```python
from build123d import *

# Parameters (mm, degrees)
F1_DEPTH = 3.175
F2_W     = 6.985
F2_H     = 3.175
F3_DEPTH = 6.35
F5_DEPTH = 25.4
F6_DEPTH = 25.4
F7_DEPTH = 26.6192
F8_DEPTH = 26.6192


# Not quite as in the source:
# - a feature names something its author has since deleted; it is built from what else it names


with BuildPart() as f1:
    # F0 (on Top) → F1 (new body)
    with BuildSketch(Plane.XY):
        Polygon((0, 63.5), (0, 0), (15.875, 0), (15.875, 12.7), (12.065, 12.7), (12.065, 50.8), (15.875, 50.8), (15.875, 63.5), align=None)
        Polygon((15.875, 12.7), (15.875, 0), (31.75, 0), (31.75, 63.5), (15.875, 63.5), (15.875, 50.8), (19.685, 50.8), (19.685, 12.7), align=None)
    extrude(amount=F1_DEPTH)

    # F2 (on face) → F3 (join)
    with BuildSketch(Plane.XZ):
        with Locations((3.4925, 1.5875)):
            Rectangle(F2_W, F2_H)
        with Locations((28.2575, 1.5875)):
            Rectangle(F2_W, F2_H)
    extrude(amount=F3_DEPTH)

    # F4 (on face) → F5 (cut)
    with BuildSketch(Plane.XY.offset(3.175)):
        with BuildLine():
            ThreePointArc((5.29375, -4.35), (3.0318335149, -3.4130835149), (3.96875, -5.675))
            Line((3.96875, -5.675), (3.96875, -4.35))
            Line((3.96875, -4.35), (5.29375, -4.35))
        make_face()
        with BuildLine():
            Line((3.96875, -4.35), (3.96875, -5.675))
            ThreePointArc((3.96875, -5.675), (4.9056664851, -5.2869164851), (5.29375, -4.35))
            Line((5.29375, -4.35), (3.96875, -4.35))
        make_face()
        with BuildLine():
            ThreePointArc((27.78125, -3.025), (26.8443335149, -3.4130835149), (26.45625, -4.35))
            Line((26.45625, -4.35), (27.78125, -4.35))
            Line((27.78125, -4.35), (27.78125, -3.025))
        make_face()
    extrude(amount=-F5_DEPTH, mode=Mode.SUBTRACT)

    # F4 (on face) → F6 (cut)
    with BuildSketch(Plane.XY.offset(3.175)):
        with BuildLine():
            ThreePointArc((29.10625, 61.5), (27.78125, 62.825), (26.45625, 61.5))
            ThreePointArc((26.45625, 61.5), (27.78125, 60.175), (29.10625, 61.5))
        make_face()
        with BuildLine():
            ThreePointArc((5.29375, 61.5), (4.9056664851, 62.4369164851), (3.96875, 62.825))
            ThreePointArc((3.96875, 62.825), (3.0318335149, 60.5630835149), (5.29375, 61.5))
        make_face()
        with BuildLine():
            Line((27.78125, -4.35), (26.45625, -4.35))
            ThreePointArc((26.45625, -4.35), (26.8443335149, -5.2869164851), (27.78125, -5.675))
            ThreePointArc((27.78125, -5.675), (28.7181664851, -5.2869164851), (29.10625, -4.35))
            ThreePointArc((29.10625, -4.35), (28.7181664851, -3.4130835149), (27.78125, -3.025))
            Line((27.78125, -3.025), (27.78125, -4.35))
        make_face()
    extrude(amount=-F6_DEPTH, mode=Mode.SUBTRACT)

    # F7 (add): a face of the model
    f7_faces = [f1.faces().sort_by_distance(p)[0] for p in [
        (31.75, 28.575, 1.5875),
    ]]
    extrude(f7_faces, amount=F7_DEPTH)

    # F8 (add): a face of the model
    f8_faces = [f1.faces().sort_by_distance(p)[0] for p in [
        (0, 28.575, 1.5875),
    ]]
    extrude(f8_faces, amount=F8_DEPTH)


solid = f1.part
```
Check sheet for the modelled part. Datum: model origin and axes. Units: mm. A direction names the side the tool comes from. Round coordinates to 2 decimals unless told otherwise and drop trailing zeros. Loops run counter-clockwise (first coordinate to the right, second up) from the corner with the lowest first, then second, coordinate; pieces in that order, holes last. Notation, with made-up numbers: (11, -5) - (20, -5) arc R20 ccw to (20, 22) - close; hole circle Ø8 at (-36.75, 38.25). An arc over 180 degrees is marked (long way). Write item = value, one per line. Start each with the question number.
Q1. Depth check by flat-ended pin: P1, Ø1, axis at x = 8, z = 1, coming from the -Y side; P2, Ø1.6, axis at x = 3.97, y = 61.5, coming from the -Z side. Enter the tip coordinate at first touch or a pass-through.
Q2. Section check C-C (z = 1.05). Record the boundary of the cut face in (x, y) (3 decimals), plus the area to 3 significant figures.
Q3. Release check for a two-part mould opening along Y. For faces 1 (the face through (16, 50.8, 2)), 2 (the face through (16, 0, 2)), 3 (the face through (27.07, 60.38, 1.61)), 4 (the face through (26, 28, 3.175)) record: pulls with the +Y half, pulls with the -Y half, needs draft (parallel to the pull), parting line crosses it, or undercut.
Q4. Thickness scan on L1, parallel to X at y = 61.5, z = 1.4; L2, parallel to Y at x = 28, z = 0.7; L3, parallel to X at y = -4.35, z = 1.1 (3 decimals). Record the ranges inside material, lowest first.
Q5. Section check B-B (x = 14.5). Record the boundary of the cut face in (y, z) (3 decimals), plus the area to 3 significant figures.
Q6. Access from +Z, -Z, +X, -X, +Y, -Y to the whole of each face (thin tool, end or side, straight path). Record for faces 5 (the face through (58.369, 28, 2)), 6 (the face through (24.765, -3, 2)), 7 (the face through (19.685, 32, 2)).
Q7. Section check A-A (y = -1). Record the boundary of the cut face in (x, z) (3 decimals), plus the area to 3 significant figures.
Derived:
q1.P1 = 0
q1.P2 = through
q2.outline = (-26.619, -6.35) - (6.985, -6.35) - (6.985, 0) - (24.765, 0) - (24.765, -6.35) - (58.369, -6.35) - (58.369, 63.5) - (-26.619, 63.5) - close; hole circle Ø2.65 at (3.969, -4.35); hole circle Ø2.65 at (3.969, 61.5); hole (12.065, 12.7) - (19.685, 12.7) - (19.685, 50.8) - (12.065, 50.8) - close; hole circle Ø2.65 at (27.781, -4.35); hole circle Ø2.65 at (27.781, 61.5)
q2.area = 5,510 mm^2
q3.face_1 = undercut
q3.face_2 = pulls with the -Y half
q3.face_3 = undercut
q3.face_4 = needs draft
q4.L1 = -26.62 to 2.64, 5.29 to 26.46, 29.11 to 58.37
q4.L2 = -6.35 to -5.66, -3.04 to 60.19, 62.81 to 63.5
q4.L3 = -26.619 to 2.644, 5.294 to 6.985, 24.765 to 26.456, 29.106 to 58.369
q5.outline = (0, 0) - (12.7, 0) - (12.7, 3.175) - (0, 3.175) - close; (50.8, 0) - (63.5, 0) - (63.5, 3.175) - (50.8, 3.175) - close
q5.area = 80.6 mm^2
q6.face_5 = +Z, -Z, +X, +Y, -Y
q6.face_6 = +Z, -Z, -Y
q6.face_7 = +Z, -Z
q7.outline = (-26.619, 0) - (6.985, 0) - (6.985, 3.175) - (-26.619, 3.175) - close; (24.765, 0) - (58.369, 0) - (58.369, 3.175) - (24.765, 3.175) - close
q7.area = 213 mm^2
